from build123d import *

# Parameters (mm, degrees)
SKETCH1_R               = 20
BOSS_EXTRUDE1_DEPTH     = 80
SKETCH2_W               = 20
SKETCH2_H               = 120
CUT_EXTRUDE1_DEPTH      = 85.852813742
FILLET1_R               = 10
CUT_EXTRUDE2_DEPTH      = 85.85281386
CUT_EXTRUDE2_DEPTH_BACK = 85.85281386
SKETCH3_R               = 7.5


with BuildPart() as part:
    # Sketch1 → Boss-Extrude1 (new body)
    with BuildSketch(Plane(origin=(0, 0, 0), x_dir=(1, 0, 0), z_dir=(0, 1, 0))):
        with Locations(Location((0, 0, 0), (0, 0, 270))):
            Circle(SKETCH1_R)
    extrude(amount=BOSS_EXTRUDE1_DEPTH)

    # Sketch2 → Cut-Extrude1 (cut, symmetric)
    with BuildSketch(Plane(origin=(0, 0, 0), x_dir=(0, 0, -1), z_dir=(1, 0, 0))):
        with Locations((-20, 80)):
            Rectangle(SKETCH2_W, SKETCH2_H)
    cut_extrude1 = extrude(amount=CUT_EXTRUDE1_DEPTH, both=True, mode=Mode.SUBTRACT)

    # Mirror1: Cut-Extrude1 across plane
    add(cut_extrude1.mirror(Plane.XY), mode=Mode.SUBTRACT)

    # Fillet1
    fillet1_edges = [part.edges().sort_by_distance(p)[0] for p in [
        (20, 80, 0),
        (-20, 80, 0),
    ]]
    fillet(fillet1_edges, radius=FILLET1_R - 0.0001)  # a hair under: the kernel refuses the full size

    # Sketch3 → Cut-Extrude2 (cut, two sides: drawn at the far end of the back side and taken through both)
    with BuildSketch(Plane.XY.offset(-CUT_EXTRUDE2_DEPTH_BACK)):
        with Locations(Location((0, 65, 0), (0, 0, 180))):
            Circle(SKETCH3_R)
    extrude(amount=CUT_EXTRUDE2_DEPTH + CUT_EXTRUDE2_DEPTH_BACK, mode=Mode.SUBTRACT)


solid = part.part
Source: CAD feature listing. Evaluate the final solid. Frame: model axes, mm. A direction names the side the tool comes from. Round coordinates to 2 decimals unless told otherwise and drop trailing zeros. Loops run counter-clockwise (first coordinate to the right, second up) from the corner with the lowest first, then second, coordinate; pieces in that order, holes last. Notation, with made-up numbers: M 59.5,-22.5 L 93.5,-22.5 A23 cw 93.5,15.5 Z; hole C 73.25,37 d9. An arc over 180 degrees is marked long. Answer as CSV lines item,"result".
Q1. Contact query for flat-ended pins moving along their axis: pin 1 (9 mm diameter, centred on x = 0, y = 65, fed in from -Z); pin 2 (1 mm diameter, centred on x = 1, y = 17, fed in from -Z); pin 3 (5 mm diameter, centred on x = 1.5, z = -17, fed in from +Y); pin 4 (10.5 mm diameter, centred on x = 8.5, y = 57, fed in from -Z). Output: stop coordinate, or through.
Verdict:
pin 1,"passes through"
pin 2,"stops at z = -19.99"
pin 3,"stops at y = 20"
pin 4,"stops at z = -10"
Q2. Pull-direction query (Y, two-part tool) for faces 4 (the face through (0, 50, -10)), 5 (the face through (0, 80, 0)), 6 (the face through (0.976, 57.564, -0.14)), 7 (the face through (0, 0, 0)); classes: +Y half, -Y half, draft (parallel to the pull), parting line (faces both ways), or undercut.
Verdict:
face 4,"draft"
face 5,"+Y half"
face 6,"undercut"
face 7,"-Y half"
Q3. Reachability of faces 1 (the face through (0, 20, -14)), 2 (the face through (-19.524, 26.732, -4.336)), 3 (the face through (0, 20, 14)) from +Z, -Z, +X, -X, +Y, -Y: full face, straight path, thin tool, end or side. Return the list, or none.
Verdict:
face 1,"-Z, +X, -X, +Y"
face 2,"+Y, -Y"
face 3,"+Z, +X, -X, +Y"
Q4. Cut plane B-B (y = 15.5). Return the cut outline in (x, z).
Verdict:
outline,"C 0,0 d40"
Q5. Line query: line 1 along Y through (x, z) = (0, 4); line 2 along Z through (x, y) = (-3, 51.5); line 3 along Y through (x, z) = (-3, -5). Output: solid intervals per line, ascending.
Verdict:
line 1,"y = 0 to 57.5, 72.5 to 80"
line 2,"z = -10 to 10"
line 3,"y = 0 to 58.13, 71.87 to 80"
Q6. Cut plane C-C (z = -11.5). Return the cut outline in (x, y).
Verdict:
outline,"M -16.36,0 L 16.36,0 L 16.36,20 L -16.36,20 Z"
Q7. Cut plane A-A (z = 0). Return the cut outline in (x, y).
Verdict:
outline,"M -20,0 L 20,0 L 20,70 A10 ccw 10,80 L -10,80 A10 ccw -20,70 Z; hole C 0,65 d15"
Q8. Cut plane D-D (y = 74). Return the cut outline in (x, z), plus the area to 3 significant figures.
Verdict:
outline,"M -16.35,-10 L 16.35,-10 A19.17 ccw 16.35,10 L -16.35,10 A19.17 ccw Z"
area,"730 mm^2"
